Design review of the part built by this model. Coordinates are the model's own, in mm. A direction names the side the tool comes from. Coordinates: 2 decimals unless noted, no trailing zeros. Loops run counter-clockwise (first coordinate to the right, second up) from the corner with the lowest first, then second, coordinate; pieces in that order, holes last. Notation, with made-up numbers: M 51.25,34 L 65.25,34 A22 cw 65.25,59 Z; hole C -38.5,30.25 d11. An arc over 180 degrees is marked long. Answer as a JSON object with one key per item and string values. Group by question number.
1. Consider section A-A (x = 4). State the section outline as (y, z) points.
2. Insertion check: pin 1 (6 mm diameter, centred on x = 1.5, z = -1.5, fed in from -Y); pin 2 (1.5 mm diameter, centred on x = 5, y = -1.5, fed in from -Z); pin 3 (5 mm diameter, centred on x = 6, z = 1, fed in from +Y). Each pin has a flat end and moves straight along its axis. Give the tip position at first contact, or say it passes through.
3. To check wall thickness, follow probe 1 along Z at (x, y) = (5.5, 0); probe 2 along X at (y, z) = (-3, 2); probe 3 along Y at (x, z) = (3, 2.75). State the ranges of each line that lie inside material, in increasing order.
4. Draft analysis for pull direction Z (two halves, no side actions). For faces 1 (the flat face through (-2.8, 1.04, -1.04)), 2 (the flat face through (-1.568, 1.088, 0.616)), 3 (the cylindrical face through (2, -3, 0)), state which applies: +Z half, -Z half, draft (parallel to the pull), parting line (faces both ways), or undercut.
5. Machinability: for faces 4 (the flat face through (0, 3.3, 0.1)), 5 (the flat face through (9.5, 0, 0)), 6 (the flat face through (-1.57, -1.08, 0.63)), which of the approach directions +Z, -Z, +X, -X, +Y, -Y give a long, thin tool a straight path to every point of the face, cutting with its end or side? Answer none if there is none.
6. Consider section B-B (z = -2.5). State the section outline as (x, y) points.
7. Consider section C-C (y = -3.25). State the section outline as (x, z) points.
Autodesk Inventor part; units mm, degrees
ref_plane "YZ Plane" through (0, 0, 0) normal (1, 0, 0) x (0, 1, 0)
ref_plane "XZ Plane" through (0, 0, 0) normal (0, 1, 0) x (-1, 0, 0)
ref_plane "XY Plane" through (0, 0, 0) normal (0, 0, 1) x (1, 0, 0)
sketch "Sketch_1" plane through (0, 0, 0) normal (0, 0, 1) x (1, 0, 0)
  line L0 (4.5, 0) -> (-2.8, 0)
  line L1 (-2.8, 0) -> (-2.8, 5)
  line L2 (-2.8, 5) -> (0, 5)
  line L3 (0, 5) -> (0, 3)
  line L4 (0, 3) -> (4.5, 3)
  line L5 (4.5, 3) -> (4.5, 0)
  line L6 (4.5, 0) -> (-2.8, 0)
revolve "Revolution1" add sketch "Sketch_1" angle 360 about axis through (4.5, 0, 0) along (1, 0, 0)
sketch "Sketch2" plane through (-2.8, 0, 0) normal (-1, 0, 0) x (0, 0, 1)
  point P0 (0, 0)
hole "Hole1" at (-2.8, 0, 0) direction (1, 0, 0) diameter 2.5 depth 2.5 tip angle 120
sketch "Sketch_3" plane through (-2.8, 0, 0) normal (1, 0, 0) x (0, 0, -1)
  line L0 (-1.25, -0.7217) -> (0, -1.4434)
  line L1 (0, -1.4434) -> (1.25, -0.7217)
  line L2 (1.25, -0.7217) -> (1.25, 0.7217)
  line L3 (1.25, 0.7217) -> (0, 1.4434)
  line L4 (0, 1.4434) -> (-1.25, 0.7217)
  line L5 (-1.25, 0.7217) -> (-1.25, -0.7217)
extrude "Extrusion1" cut sketch "Sketch_3" along normal blind 2.5
sketch "Sketch_6" plane through (0, 0, 0) normal (0, 0, 1) x (1, 0, 0)
  line L0 (9.5, 0) -> (4.5, 0)
  line L1 (4.5, 0) -> (4.5, 2)
  line L2 (4.5, 2) -> (9.0705, 2)
  line L3 (9.0705, 2) -> (9.5, 1.5705)
  line L4 (9.5, 1.5705) -> (9.5, 0)
  line L5 (9.5, 0) -> (4.5, 0)
revolve "Revolution2" add sketch "Sketch_6" angle 360 about axis through (9.5, 0, 0) along (1, 0, 0)
thread "Thread1"
properties part number "DBTS4-4.5-5-LTC"
Findings below:
{
 "1": {"outline": "C 0,0 d6"},
 "2": {"pin 1": "stops at y = -5", "pin 2": "stops at z = -2.85", "pin 3": "stops at y = 3"},
 "3": {"probe 1": "z = -2 to 2", "probe 2": "x = -2.8 to 0", "probe 3": "y = -1.2 to 1.2"},
 "4": {"face 1": "draft", "face 2": "undercut", "face 3": "parting line"},
 "5": {"face 4": "+X", "face 5": "+Z, -Z, +X, +Y, -Y", "face 6": "-X"},
 "6": {"outline": "M -2.8,-4.33 L 0,-4.33 L 0,-1.66 L 4.5,-1.66 L 4.5,1.66 L 0,1.66 L 0,4.33 L -2.8,4.33 Z"},
 "7": {"outline": "M -2.8,-3.8 L 0,-3.8 L 0,3.8 L -2.8,3.8 Z"}
}
